Input: part model. Units: mm. Frame: model coordinates. Give positions to 0.01 mm unless a question says otherwise; leave off trailing zeros. Write each loop counter-clockwise with the first axis right and the second up, starting at its lowest first coordinate (ties: lowest second). Pieces come first, ordered by that corner, then holes. Notation, with made-up numbers: (15, 6.5) -> (70, 6.5) arc R21 cw to (70, 30.5) -> close; hole circle Ø5 at (38, 52). An arc over 180 degrees is marked (long way). Answer as a JSON object with one key per item and string values. Group by question number.
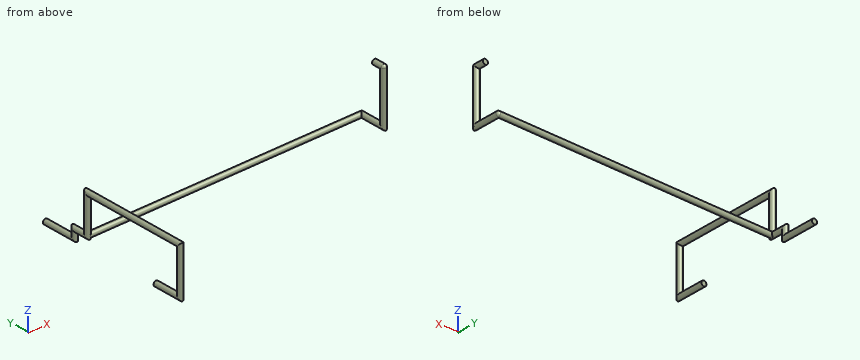
from build123d import *

# Parameters (mm, degrees)
F0_R  = 7.5
F3_R  = 7.5
F7_R  = 7.5
F11_R = 7.5


with BuildPart() as f2:
    # F2: sweep along a path in F1
    with BuildLine(Plane.YZ) as f2_path:
        Line((0, 0), (-80.781, 0))
        Line((-80.781, 0), (-80.781, 134.381))
        Line((-80.781, 134.381), (228, 134.381))
        Line((228, 134.381), (228, 24.381))
        Line((228, 24.381), (270.740032196, 24.381))
        Line((270.740032196, 24.381), (270.740032196, 0))
        Line((270.740032196, 0), (367.740032196, 0))
    # F0 (on Front) → F2 (sweep)
    with BuildSketch(Plane.XZ):
        Circle(F0_R)
    sweep(path=f2_path.line, transition=Transition.RIGHT)

    # F5: sweep along a path in F4
    with BuildLine(Plane.XZ) as f5_path:
        Line((0, 0), (810.75, 0))
    # F3 (on Right) → F5 (sweep)
    with BuildSketch(Plane.YZ):
        with Locations((228, 24.381)):
            Circle(F3_R)
    sweep(path=f5_path.line)

    # F9: sweep along a path in F8
    with BuildLine(Plane.YZ) as f9_path:
        Line((228, 24.381), (154.713, 24.381))
        Line((154.713, 24.381), (154.713, 176.355))
    # F7 (on offset) → F9 (sweep)
    with BuildSketch(Plane.XZ.offset(-228)):
        with Locations((810.75, 24.381)):
            Circle(F7_R)
    sweep(path=f9_path.line, transition=Transition.RIGHT)

    # F9_face (on face) → F13 (revolve)
    with BuildSketch(Plane(origin=(813.9330988618, 228, 24.381), x_dir=(-1, 0, 0), z_dir=(0, 1, 0))):
        with BuildLine():
            ThreePointArc((-4.3169011382, 0), (-2.1202019971, -5.3033008589), (3.1830988618, -7.5))
            Line((3.1830988618, -7.5), (3.1830988618, 7.5))
            ThreePointArc((3.1830988618, 7.5), (-2.1202019971, 5.3033008589), (-4.3169011382, 0))
        make_face()
    revolve(axis=Axis((810.75, 228, 24.381), (0, 0, 1)))

    # F14: sweep along a path in F12
    with BuildLine(Plane.XY) as f14_path:
        Line((862, 154.713), (862, 184.713))
    # F11 (on offset) → F14 (sweep)
    with BuildSketch(Plane.XZ.offset(-154.713)):
        with Locations((810.75, 176.355)):
            Circle(F11_R)
    sweep(path=f14_path.line)

    # F9_face1 (on face) → F15 (revolve)
    with BuildSketch(Plane(origin=(810.75, 151.5299011382, 176.355), x_dir=(1, 0, 0), z_dir=(0, 0, 1))):
        with BuildLine():
            ThreePointArc((-7.5, 3.1830988618), (0, -4.3169011382), (7.5, 3.1830988618))
            Line((7.5, 3.1830988618), (-7.5, 3.1830988618))
        make_face()
    revolve(axis=Axis((810.75, 154.713, 176.355), (1, 0, 0)))


solid = f2.part
1. Section A-A (y = -36.5). Return the cut outline in (x, z), plus the area to 3 significant figures.
2. Contact query for flat-ended pins moving along their axis: pin 1 Ø5 at (y, z) = (143.5, 151.5) entering from +X; pin 2 Ø4.5 at (x, z) = (808, 177.5) entering from +Y; pin 3 Ø10 at (x, z) = (588, 30.5) entering from -Y. Output: stop coordinate, or through.
3. Section D-D (x = 239). Return the cut outline in (y, z), plus the area to 3 significant figures.
4. Section B-B (z = 96.5). Return the cut outline in (x, y).
5. Section C-C (y = 322.5). Return the cut outline in (x, z), plus the area to 3 significant figures.
6. Line query: line 1 (Z direction, x = 96, y = 231); line 2 (Y direction, x = 196.5, z = 29). Output: solid intervals per line, ascending.
Working result:
{
 "1": {"outline": "circle Ø15 at (0, 0); circle Ø15 at (0, 134.38)", "area": "353 mm^2"},
 "2": {"pin 1": "passes through", "pin 2": "stops at y = 184.71", "pin 3": "stops at y = 220.58"},
 "3": {"outline": "circle Ø15 at (228, 24.38)", "area": "177 mm^2"},
 "4": {"outline": "circle Ø15 at (0, -80.78); circle Ø15 at (0, 228); circle Ø15 at (810.75, 154.71)"},
 "5": {"outline": "circle Ø15 at (0, 0)", "area": "177 mm^2"},
 "6": {"line 1": "z = 17.51 to 31.25", "line 2": "y = 222.09 to 233.91"}
}
